Part model, mm, in its own coordinate system. Face numbers are marked on the shaded views. A direction names the side the tool comes from. Give positions to 0.01 mm unless a question says otherwise; leave off trailing zeros. Write each loop counter-clockwise with the first axis right and the second up, starting at its lowest first coordinate (ties: lowest second). Pieces come first, ordered by that corner, then holes. Notation, with made-up numbers: M 49,-20.5 L 55,-20.5 A17 ccw 55,-2.5 Z; hole C -16.5,55.25 d6. An arc over 180 degrees is marked long. Use CSV: the item, a comma, the result in double quotes. Start each with the question number.
1. Band-saw the part on C-C, the plane y = -1. List the corners of the cut face in (x, z).
2. Band-saw the part on D-D, the plane y = 5.5. List the corners of the cut face in (x, z), then the cut area to 3 significant figures.
3. Band-saw the part on A-A, the plane z = 0. List the corners of the cut face in (x, y), then the cut area to 3 significant figures.
4. Drill centre lines: line 1 along Y through (x, z) = (-5.5, 2.25); line 2 along Y through (x, z) = (-5.5, 4.5); line 3 along Z through (x, y) = (4.5, 7). Where is each one in solid material? Low to high. Write a range as from..to.
5. Band-saw the part on B-B, the plane x = 0. List the corners of the cut face in (y, z).
6. Drop flat-ended pins along their axis: pin 1 Ø1.5 at (x, y) = (4, 1) entering from +Z; pin 2 Ø2 at (y, z) = (-0.5, -3.5) entering from -X; pin 3 Ø2 at (y, z) = (7, -3.5) entering from +X. Give the stop position or say it passes through.
7. 3-axis set-ups, long thin cutter, end or side, ignore diameter. For the marked faces 1, 2 and 3: which of +Z, -Z, +X, -X, +Y, -Y reach the whole face in a straight line?
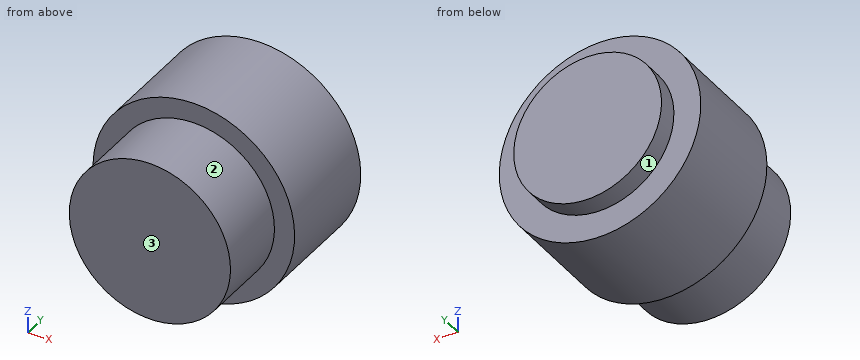
from build123d import *

# Parameters (mm, degrees)
THREAD_START        = -3.5
SKETCH1_R           = 6
THREAD_DEPTH        = 5.33
BODY_START          = 1.82
SKETCH2_R           = 7.5
BODY_DEPTH          = 8
FRONT_START         = 9.81
SKETCH3_R           = 5.5
FRONT_ELEMENT_DEPTH = 1.51


with BuildPart() as part:
    # Sketch1 → Thread (new body)
    with BuildSketch(Plane(origin=(0, 0, 0), x_dir=(1, 0, 0), z_dir=(0, 1, 0)).offset(THREAD_START)):
        with Locations(Location((0, 0, 0), (0, 0, 270))):
            Circle(SKETCH1_R)
    extrude(amount=THREAD_DEPTH)

    # Sketch2 → Body (add)
    with BuildSketch(Plane(origin=(0, 0, 0), x_dir=(1, 0, 0), z_dir=(0, 1, 0)).offset(BODY_START)):
        with Locations(Location((0, 0, 0), (0, 0, 270))):
            Circle(SKETCH2_R)
    extrude(amount=BODY_DEPTH)

    # Sketch3 → Front element (add)
    with BuildSketch(Plane(origin=(0, 0, 0), x_dir=(1, 0, 0), z_dir=(0, 1, 0)).offset(FRONT_START)):
        with Locations(Location((0, 0, 0), (0, 0, 270))):
            Circle(SKETCH3_R)
    extrude(amount=FRONT_ELEMENT_DEPTH)


solid = part.part
Output:
1,outline,"C 0,0 d12"
2,outline,"C 0,0 d15"
2,area,"177 mm²"
3,outline,"M -7.5,1.82 L -6,1.82 L -6,-3.5 L 6,-3.5 L 6,1.82 L 7.5,1.82 L 7.5,9.82 L 5.5,9.82 L 5.5,11.32 L -5.5,11.32 L -5.5,9.82 L -7.5,9.82 Z"
3,area,"200 mm²"
4,line 1,"y = -3.5..9.82"
4,line 2,"y = 1.82..9.82"
4,line 3,"z = -6..6"
5,outline,"M -3.5,-6 L 1.82,-6 L 1.82,-7.5 L 9.82,-7.5 L 9.82,-5.5 L 11.32,-5.5 L 11.32,5.5 L 9.82,5.5 L 9.82,7.5 L 1.82,7.5 L 1.82,6 L -3.5,6 Z"
6,pin 1,"stops at z = 5.04"
6,pin 2,"stops at x = -5.45"
6,pin 3,"stops at x = 7.07"
7,face 1,"+Y"
7,face 2,"-Y"
7,face 3,"+Z, -Z, +X, -X, -Y"
